from build123d import *
from OCP.BRepFilletAPI import BRepFilletAPI_MakeChamfer

# Parameters (mm, degrees)
SKETCH_1_W          = 95
SKETCH_1_H          = 120
EXTRUDE_1_DEPTH     = 3
SKETCH_2_W          = 3
SKETCH_2_H          = 37.7
EXTRUDE_2_DEPTH     = 70
SKETCH_4_R          = 1.5
CUT_EXTRUDE_2_DEPTH = 10
SKETCH_18_W         = 5
SKETCH_18_H         = 12
CUT_EXTRUDE_5_DEPTH = 20
SKETCH_21_R         = 1.65
CUT_EXTRUDE_6_DEPTH = 10
SKETCH_22_R         = 1.56
CUT_EXTRUDE_7_DEPTH = 10
SKETCH_3_R          = 2.125
CUT_EXTRUDE_8_DEPTH = 80
SKETCH_23_W         = 41.335758236
SKETCH_23_H         = 27
CUT_EXTRUDE_9_DEPTH = 80
CHAMFER_4_SIZE      = 3
CHAMFER_4_SIZE2     = 6.433520762
CHAMFER_5_SIZE      = 5
CHAMFER_5_SIZE2     = 2.331538291
SKETCH_24_W         = 15
SKETCH_24_H         = 3.5
EXTRUDE_3_DEPTH     = 64
CHAMFER_7_SIZE      = 5
SKETCH_26_W         = 64
SKETCH_26_H         = 4
EXTRUDE_5_DEPTH     = 8
SKETCH_5_W          = 64
SKETCH_5_H          = 4
EXTRUDE_6_DEPTH     = 5
CHAMFER_9_SIZE      = 2


with BuildPart() as part:
    # 草图1 → 凸台-拉伸1 (new body)
    with BuildSketch(Plane.XY):
        Rectangle(SKETCH_1_W, SKETCH_1_H)
    extrude(amount=EXTRUDE_1_DEPTH)

    # 草图2 → 凸台-拉伸2 (add)
    with BuildSketch(Plane(origin=(0, 0, 0), x_dir=(-1, 0, 0), z_dir=(0, 0, -1))):
        with Locations((-33.5, 0)):
            Rectangle(SKETCH_2_W, SKETCH_2_H)
        with Locations((33.5, 0)):
            Rectangle(SKETCH_2_W, SKETCH_2_H)
    extrude(amount=EXTRUDE_2_DEPTH)

    # 草图4 → 切除-拉伸2 (cut)
    with BuildSketch(Plane.XY.offset(3)):
        with Locations((-32.5, 57)):
            Circle(SKETCH_4_R)
        with Locations(Location((32.5, 57, 0), (0, 0, 180))):
            Circle(SKETCH_4_R)
        with Locations((32.5, -57)):
            Circle(SKETCH_4_R)
        with Locations(Location((-32.5, -57, 0), (0, 0, 180))):
            Circle(SKETCH_4_R)
    extrude(amount=-CUT_EXTRUDE_2_DEPTH, mode=Mode.SUBTRACT)

    # 草图18 → 切除-拉伸5 (cut)
    with BuildSketch(Plane.XY.offset(3)):
        with Locations((-17.5, -26)):
            Rectangle(SKETCH_18_W, SKETCH_18_H)
        with Locations((17.5, -26)):
            Rectangle(SKETCH_18_W, SKETCH_18_H)
        with Locations((-17.5, -46)):
            Rectangle(SKETCH_18_W, SKETCH_18_H)
        with Locations((17.5, -46)):
            Rectangle(SKETCH_18_W, SKETCH_18_H)
        with Locations((17.5, 46)):
            Rectangle(SKETCH_18_W, SKETCH_18_H)
        with Locations((-17.5, 46)):
            Rectangle(SKETCH_18_W, SKETCH_18_H)
        with Locations((17.5, 26)):
            Rectangle(SKETCH_18_W, SKETCH_18_H)
        with Locations((-17.5, 26)):
            Rectangle(SKETCH_18_W, SKETCH_18_H)
    extrude(amount=-CUT_EXTRUDE_5_DEPTH, mode=Mode.SUBTRACT)

    # 草图21 → 切除-拉伸6 (cut)
    with BuildSketch(Plane.XY.offset(3)):
        with Locations((-35.5, -48)):
            Circle(SKETCH_21_R)
        with Locations((-35.5, -30)):
            Circle(SKETCH_21_R)
        with Locations(Location((35.5, -30, 0), (0, 0, 180))):
            Circle(SKETCH_21_R)
        with Locations(Location((35.5, -48, 0), (0, 0, 180))):
            Circle(SKETCH_21_R)
        with Locations((35.5, 48)):
            Circle(SKETCH_21_R)
        with Locations((35.5, 30)):
            Circle(SKETCH_21_R)
        with Locations(Location((-35.5, 30, 0), (0, 0, 180))):
            Circle(SKETCH_21_R)
        with Locations(Location((-35.5, 48, 0), (0, 0, 180))):
            Circle(SKETCH_21_R)
    extrude(amount=-CUT_EXTRUDE_6_DEPTH, mode=Mode.SUBTRACT)

    # 草图22 → 切除-拉伸7 (cut)
    with BuildSketch(Plane.XY.offset(3)):
        with Locations((-7.78, -55)):
            Circle(SKETCH_22_R)
        with Locations(Location((7.78, -55, 0), (0, 0, 180))):
            Circle(SKETCH_22_R)
        with Locations((7.78, 55)):
            Circle(SKETCH_22_R)
        with Locations(Location((-7.78, 55, 0), (0, 0, 180))):
            Circle(SKETCH_22_R)
    extrude(amount=-CUT_EXTRUDE_7_DEPTH, mode=Mode.SUBTRACT)

    # 草图3 → 切除-拉伸8 (cut)
    with BuildSketch(Plane(origin=(35, 0, 0), x_dir=(0, 0, -1), z_dir=(1, 0, 0))):
        with Locations((13, -1)):
            Circle(SKETCH_3_R)
        with Locations((13, -10.85)):
            Circle(SKETCH_3_R)
        with Locations((62.42, -1)):
            Circle(SKETCH_3_R)
        with Locations((62.42, -10.85)):
            Circle(SKETCH_3_R)
    extrude(amount=-CUT_EXTRUDE_8_DEPTH, mode=Mode.SUBTRACT)

    # 草图23 → 切除-拉伸9 (cut)
    with BuildSketch(Plane(origin=(35, 0, 0), x_dir=(0, 0, -1), z_dir=(1, 0, 0))):
        with Locations((37.71, -5.35)):
            Rectangle(SKETCH_23_W, SKETCH_23_H)
    extrude(amount=-CUT_EXTRUDE_9_DEPTH, mode=Mode.SUBTRACT)

    # 倒角4: one chamfer whose edges measure the first distance from different faces: ONE call of the kernel's chamfer builder (chamfer() names one face for all edges)
    chamfer_4_edges_1 = [part.edges().sort_by_distance(p)[0] for p in [
        (-33.5, 8.15, -58.377879118),
    ]]
    chamfer_4_side_1 = [part.faces().sort_by_distance(p)[0] for p in [
        (-33.5, -5.35, -58.377879118),
    ]]
    chamfer_4_edges_2 = [part.edges().sort_by_distance(p)[0] for p in [
        (33.5, 8.15, -58.377879118),
    ]]
    chamfer_4_side_2 = [part.faces().sort_by_distance(p)[0] for p in [
        (33.5, -5.35, -58.377879118),
    ]]
    chamfer_4 = BRepFilletAPI_MakeChamfer(part.part.solid().wrapped)
    for e in chamfer_4_edges_1:
        chamfer_4.Add(CHAMFER_4_SIZE, CHAMFER_4_SIZE2, e.wrapped, chamfer_4_side_1[0].wrapped)  # the first distance lies on this face
    for e in chamfer_4_edges_2:
        chamfer_4.Add(CHAMFER_4_SIZE, CHAMFER_4_SIZE2, e.wrapped, chamfer_4_side_2[0].wrapped)  # the first distance lies on this face
    add(Compound.cast(chamfer_4.Shape()), mode=Mode.REPLACE)

    # 倒角5: one chamfer whose edges measure the first distance from different faces: ONE call of the kernel's chamfer builder (chamfer() names one face for all edges)
    chamfer_5_edges_1 = [part.edges().sort_by_distance(p)[0] for p in [
        (-33.5, 8.15, -17.042120882),
    ]]
    chamfer_5_side_1 = [part.faces().sort_by_distance(p)[0] for p in [
        (-33.5, 8.15, -34.493239619),
    ]]
    chamfer_5_edges_2 = [part.edges().sort_by_distance(p)[0] for p in [
        (33.5, 8.15, -17.042120882),
    ]]
    chamfer_5_side_2 = [part.faces().sort_by_distance(p)[0] for p in [
        (33.5, 8.15, -34.493239619),
    ]]
    chamfer_5 = BRepFilletAPI_MakeChamfer(part.part.solid().wrapped)
    for e in chamfer_5_edges_1:
        chamfer_5.Add(CHAMFER_5_SIZE, CHAMFER_5_SIZE2, e.wrapped, chamfer_5_side_1[0].wrapped)  # the first distance lies on this face
    for e in chamfer_5_edges_2:
        chamfer_5.Add(CHAMFER_5_SIZE, CHAMFER_5_SIZE2, e.wrapped, chamfer_5_side_2[0].wrapped)  # the first distance lies on this face
    add(Compound.cast(chamfer_5.Shape()), mode=Mode.REPLACE)

    # 草图24 → 凸台-拉伸3 (add)
    with BuildSketch(Plane(origin=(-32, 0, 0), x_dir=(0, 0, -1), z_dir=(1, 0, 0))):
        with Locations((7.5, 17.1)):
            Rectangle(SKETCH_24_W, SKETCH_24_H)
        with Locations((62.5, 17.1)):
            Rectangle(SKETCH_24_W, SKETCH_24_H)
    extrude(amount=EXTRUDE_3_DEPTH)

    # 倒角7
    chamfer_7_edges = [part.edges().sort_by_distance(p)[0] for p in [
        (-32, 17.1, -15),
        (32, 17.1, -15),
        (-32, 17.1, -55),
        (32, 17.1, -55),
    ]]
    chamfer(chamfer_7_edges, length=CHAMFER_7_SIZE)

    # 草图26 → 凸台-拉伸5 (add)
    with BuildSketch(Plane(origin=(0, 0, 0), x_dir=(-1, 0, 0), z_dir=(0, 0, -1))):
        with Locations((0, -16.85)):
            Rectangle(SKETCH_26_W, SKETCH_26_H)
    extrude(amount=EXTRUDE_5_DEPTH)

    # 草图5 → 凸台-拉伸6 (add)
    with BuildSketch(Plane(origin=(0, 0, -70), x_dir=(-1, 0, 0), z_dir=(0, 0, -1))):
        with Locations((0, -16.85)):
            Rectangle(SKETCH_5_W, SKETCH_5_H)
    extrude(amount=-EXTRUDE_6_DEPTH)

    # 倒角9
    chamfer_9_edges = [part.edges().sort_by_distance(p)[0] for p in [
        (0, -14.85, -65),
    ]]
    chamfer(chamfer_9_edges, length=CHAMFER_9_SIZE)


solid = part.part
Verification items for the finished model (mm, model axes). A direction names the side the tool comes from. Coordinates: 2 decimals unless noted, no trailing zeros. Order: outer loops, then holes, each group sorted by start corner. A loop starts at its lowest first (then second) coordinate and runs counter-clockwise, first axis right, second up. Notation, with made-up numbers: (19.25, -38) -> (36.25, -38) arc R26 ccw to (36.25, -13) -> close; hole circle Ø7 at (-13.75, 46.5). An arc over 180 degrees is marked (long way). Put each result on its own line as item: value. Start each with the question number.
1. Cross-section at C-C, the plane y = 48. Record the boundary of the cut face in (x, z).
2. Cross-section at D-D, the plane z = -13. Record the boundary of the cut face in (x, y) (3 decimals), then the cut area to 3 significant figures.
3. Access from +Z, -Z, +X, -X, +Y, -Y to the whole of each face (thin tool, end or side, straight path). Record for faces 1 (the flat face through (-20, -26, 2)), 2 (the flat face through (-33.48, 6.97, -19.51)), 3 (the flat face through (0, -18.85, -3)), 4 (the flat face through (0, 18.85, -11)).
4. Mould release check, pull along Z, two halves, no side actions. Record for faces 5 (the flat face through (-35, 12, -35)), 6 (the flat face through (33.52, 6.67, -55.12)): released by +Z, released by -Z, zero draft, split by the parting line, or undercut.
5. Material ranges on L1, parallel to Y at x = -18.5, z = -7; L2, parallel to Y at x = -35, z = 1; L3, parallel to Z at x = 15, y = 16, recorded low to high. Write a range as [from, to].
6. Go/stop test with flat-tipped pins: pin 1 Ø2.5 at (x, y) = (-35.5, 48) entering from +Z; pin 2 Ø5.5 at (x, y) = (35.5, -30) entering from -Z; pin 3 Ø8 at (x, z) = (-15, -18.5) entering from -Y; pin 4 Ø1.5 at (y, z) = (11, -59.5) entering from +X. Record where each tip stops, or that it passes through.
7. Cross-section at A-A, the plane x = -7.78. Count the separate pieces of the cut face and the enclosed holes in it, then the cut area to 3 significant figures.
8. Cross-section at B-B, the plane z = -27.5. Record the boundary of the cut face in (x, y).
Computed:
1. outline: (-47.5, 0) -> (-37.15, 0) -> (-37.15, 3) -> (-47.5, 3) -> close; (-33.85, 0) -> (-20, 0) -> (-20, 3) -> (-33.85, 3) -> close; (-15, 0) -> (15, 0) -> (15, 3) -> (-15, 3) -> close; (20, 0) -> (33.85, 0) -> (33.85, 3) -> (20, 3) -> close; (37.15, 0) -> (47.5, 0) -> (47.5, 3) -> (37.15, 3) -> close
2. outline: (-35, -18.85) -> (-32, -18.85) -> (-32, -12.975) -> (-35, -12.975) -> close; (-35, -8.725) -> (-32, -8.725) -> (-32, -3.125) -> (-35, -3.125) -> close; (-35, 1.125) -> (-32, 1.125) -> (-32, 15.35) -> (32, 15.35) -> (32, 1.125) -> (35, 1.125) -> (35, 18.85) -> (-35, 18.85) -> close; (32, -18.85) -> (35, -18.85) -> (35, -12.975) -> (32, -12.975) -> close; (32, -8.725) -> (35, -8.725) -> (35, -3.125) -> (32, -3.125) -> close
2. area: 399 mm2
3. face 1: +Z, -Z
3. face 2: +X, -X, -Y
3. face 3: -Z, +X, -X, -Y
3. face 4: -Z, +X, -X, +Y
4. face 5: zero draft
4. face 6: undercut
5. L1: [-18.85, -14.85], [15.35, 18.85]
5. L2: [-60, -49.57], [-46.43, -31.57], [-28.43, 28.43], [31.57, 46.43], [49.57, 60]
5. L3: [-70, -55], [-15, 3]
6. pin 1: through
6. pin 2: z = 0
6. pin 3: y = 15.35
6. pin 4: x = 35
7. separate pieces: 5
7. enclosed holes: 0
7. area: 496 mm2
8. outline: (-35, 8.15) -> (-32, 8.15) -> (-32, 18.85) -> (-35, 18.85) -> close; (32, 8.15) -> (35, 8.15) -> (35, 18.85) -> (32, 18.85) -> close
